Geometry: final body of the model. Coordinates: model frame, mm. A direction names the side the tool comes from. Give positions to 0.01 mm unless a question says otherwise; leave off trailing zeros. Write each loop counter-clockwise with the first axis right and the second up, starting at its lowest first coordinate (ties: lowest second). Pieces come first, ordered by that corner, then holes. Notation, with made-up numbers: (-7, 28) -> (23, 28) arc R35 ccw to (23, 62) -> close; hole circle Ø1 at (79.5, 1.25). An arc over 180 degrees is marked (long way). Answer as a JSON object with one key per item and string values.
from build123d import *

# Parameters (mm, degrees)
BOSS_EXTRUDE1_DEPTH      = 11
SKETCH2_W                = 60
SKETCH2_H                = 5
BOSS_EXTRUDE2_DEPTH      = 26
FILLET1_R                = 5
SKETCH4_R                = 1.75
CUT_EXTRUDE2_DEPTH       = 25
CUT_EXTRUDE3_DEPTH       = 25
FILLET1_OF_MIRROR1_R     = 5
CUT_EXTRUDE7_DEPTH       = 0.5
BOSS_EXTRUDE3_DEPTH      = 10
SKETCH20_R               = 1.95
CUT_EXTRUDE10_DEPTH      = 14
FILLET2_R                = 2
SKETCH21_W               = 5
SKETCH21_H               = 13
BOSS_EXTRUDE4_DEPTH      = 10
FILLET3_R                = 2
FILLET4_R                = 2
SKETCH24_W               = 27.361524014
SKETCH24_H               = 13
CUT_EXTRUDE12_DEPTH      = 5
SKETCH22_R               = 2.25
CUT_EXTRUDE11_DEPTH      = 38.361524014
CUT_EXTRUDE11_DEPTH_BACK = 3
SKETCH23_R               = 5.5
CUT_EXTRUDE13_DEPTH      = 5
BOSS_EXTRUDE5_DEPTH      = 3
FILLET5_R                = 2


with BuildPart() as part:
    # Sketch1 → Boss-Extrude1 (new body)
    with BuildSketch(Plane.XY):
        with BuildLine():
            Line((60, 35), (0, 35))
            Line((0, 35), (0, 40))
            ThreePointArc((0, 40), (-7.071067812, 37.071067812), (-10, 30))
            Line((-10, 30), (-10, 10))
            ThreePointArc((-10, 10), (-7.071067812, 2.928932188), (0, 0))
            Line((0, 0), (60, 0))
            ThreePointArc((60, 0), (67.071067812, 2.928932188), (70, 10))
            Line((70, 10), (70, 30))
            ThreePointArc((70, 30), (67.071067812, 37.071067812), (60, 40))
            Line((60, 40), (60, 35))
        make_face()
    extrude(amount=BOSS_EXTRUDE1_DEPTH)

    # Sketch2 → Boss-Extrude2 (add)
    with BuildSketch(Plane.XY.offset(11)):
        with Locations((30, 37.5)):
            Rectangle(SKETCH2_W, SKETCH2_H)
    boss_extrude2 = extrude(amount=-BOSS_EXTRUDE2_DEPTH)

    # Fillet1
    fillet1_edges = [part.edges().sort_by_distance(p)[0] for p in [
        (0, 37.5, -15),
        (60, 37.5, -15),
    ]]
    fillet(fillet1_edges, radius=FILLET1_R)

    # Sketch4 → Cut-Extrude2 (cut)
    with BuildSketch(Plane(origin=(0, 35, 0), x_dir=(-1, 0, 0), z_dir=(0, -1, 0))):
        with Locations((-55, 7.5)):
            Circle(SKETCH4_R)
        with Locations((-30, 7.5)):
            Circle(SKETCH4_R)
        with Locations((-5, 7.5)):
            Circle(SKETCH4_R)
    cut_extrude2 = extrude(amount=-CUT_EXTRUDE2_DEPTH, mode=Mode.SUBTRACT)

    # Sketch5 → Cut-Extrude3 (cut)
    with BuildSketch(Plane.XZ.offset(-35)):
        with BuildLine():
            Line((5, -14.75), (55, -14.75))
            ThreePointArc((55, -14.75), (58.358757211, -13.358757211), (59.75, -10))
            Line((59.75, -10), (59.75, -0.25))
            Line((59.75, -0.25), (59.75, 0))
            Line((59.75, 0), (60, 0))
            Line((60, 0), (60, -10))
            ThreePointArc((60, -10), (58.535533906, -13.535533906), (55, -15))
            Line((55, -15), (5, -15))
            ThreePointArc((5, -15), (1.464466094, -13.535533906), (0, -10))
            Line((0, -10), (0, 0))
            Line((0, 0), (0.25, 0))
            Line((0.25, 0), (0.25, -0.25))
            Line((0.25, -0.25), (0.25, -10))
            ThreePointArc((0.25, -10), (1.641242789, -13.358757211), (5, -14.75))
        make_face()
    extrude(amount=-CUT_EXTRUDE3_DEPTH, mode=Mode.SUBTRACT)

    # Mirror1: Boss-Extrude2, Cut-Extrude2 across plane
    add(boss_extrude2.mirror(Plane(origin=(0, 20, 0), x_dir=(0, 0, 1), z_dir=(0, -1, 0))))
    add(cut_extrude2.mirror(Plane(origin=(0, 20, 0), x_dir=(0, 0, 1), z_dir=(0, -1, 0))), mode=Mode.SUBTRACT)

    # Fillet1 of Mirror1
    fillet1_of_mirror1_edges = [part.edges().sort_by_distance(p)[0] for p in [
        (0, 2.5, -15),
        (60, 2.5, -15),
    ]]
    fillet(fillet1_of_mirror1_edges, radius=FILLET1_OF_MIRROR1_R)

    # Sketch16 → Cut-Extrude7 (cut)
    with BuildSketch(Plane.XZ.offset(-35)):
        with BuildLine():
            Line((0.25, 0), (0.25, -10))
            ThreePointArc((0.25, -10), (1.641242789, -13.358757211), (5, -14.75))
            Line((5, -14.75), (55, -14.75))
            ThreePointArc((55, -14.75), (58.358757211, -13.358757211), (59.75, -10))
            Line((59.75, -10), (59.75, 0))
            Line((59.75, 0), (0.25, 0))
        make_face()
    extrude(amount=-CUT_EXTRUDE7_DEPTH, mode=Mode.SUBTRACT)

    # Sketch19 → Boss-Extrude3 (add)
    with BuildSketch(Plane.XY.offset(11)):
        with BuildLine():
            Line((-10, 13), (15, 13))
            Line((15, 13), (15, 9.995431427))
            ThreePointArc((15, 9.995431427), (14.414213562, 8.581217864), (13, 7.995431427))
            Line((13, 7.995431427), (0, 7.995431427))
            Line((0, 7.995431427), (0, 5.995431427))
            Line((0, 5.995431427), (15, 5.995431427))
            ThreePointArc((15, 5.995431427), (16.414213562, 6.581217864), (17, 7.995431427))
            Line((17, 7.995431427), (17, 13))
            Line((17, 13), (22, 13))
            Line((22, 13), (22, 0))
            Line((22, 0), (0, 0))
            ThreePointArc((0, 0), (-7.071067812, 2.928932188), (-10, 10))
            Line((-10, 10), (-10, 13))
        make_face()
    extrude(amount=BOSS_EXTRUDE3_DEPTH)

    # Sketch20 → Cut-Extrude10 (cut)
    with BuildSketch(Plane(origin=(0, 0, 0), x_dir=(-1, 0, 0), z_dir=(0, -1, 0))):
        with Locations((-8.068741, -16)):
            Circle(SKETCH20_R)
    extrude(amount=-CUT_EXTRUDE10_DEPTH, mode=Mode.SUBTRACT)

    # Fillet2
    fillet2_edges = [part.edges().sort_by_distance(p)[0] for p in [
        (15, 13, 16),
    ]]
    fillet(fillet2_edges, radius=FILLET2_R)

    # Sketch21 → Boss-Extrude4 (add)
    with BuildSketch(Plane.XY.offset(11)):
        with BuildLine():
            Line((70, 13), (60, 13))
            Line((60, 13), (60, 0))
            ThreePointArc((60, 0), (67.071067812, 2.928932188), (70, 10))
            Line((70, 10), (70, 13))
        make_face()
        with Locations((30.138475986, 6.5)):
            Rectangle(SKETCH21_W, SKETCH21_H)
    extrude(amount=BOSS_EXTRUDE4_DEPTH)

    # Fillet3
    fillet3_edges = [part.edges().sort_by_distance(p)[0] for p in [
        (27.638475986, 13, 16),
    ]]
    fillet(fillet3_edges, radius=FILLET3_R)

    # Fillet4
    fillet4_edges = [part.edges().sort_by_distance(p)[0] for p in [
        (27.638475986, 0, 16),
    ]]
    fillet(fillet4_edges, radius=FILLET4_R)

    # Sketch24 → Cut-Extrude12 (cut)
    with BuildSketch(Plane.XY.offset(11)):
        with Locations((46.319237993, 6.5)):
            Rectangle(SKETCH24_W, SKETCH24_H)
    extrude(amount=-CUT_EXTRUDE12_DEPTH, mode=Mode.SUBTRACT)

    # Sketch22 → Cut-Extrude11 (cut, two sides)
    with BuildSketch(Plane(origin=(32.638475986, 0, 0), x_dir=(0, 0, -1), z_dir=(1, 0, 0))) as cut_extrude11_sk:
        with Locations((-12, 6.5)):
            Circle(SKETCH22_R)
    extrude(amount=CUT_EXTRUDE11_DEPTH, mode=Mode.SUBTRACT)
    extrude(cut_extrude11_sk.sketch, amount=-CUT_EXTRUDE11_DEPTH_BACK, mode=Mode.SUBTRACT)

    # Sketch23 → Cut-Extrude13 (cut)
    with BuildSketch(Plane(origin=(70, 0, 0), x_dir=(0, 0, -1), z_dir=(1, 0, 0))):
        with Locations((-12, 6.5)):
            Circle(SKETCH23_R)
    extrude(amount=-CUT_EXTRUDE13_DEPTH, mode=Mode.SUBTRACT)

    # Sketch25 → Boss-Extrude5 (add)
    with BuildSketch(Plane.XY.offset(21)):
        with BuildLine():
            Line((60, 0), (32.638475986, 0))
            Line((32.638475986, 0), (29.638475986, 0))
            ThreePointArc((29.638475986, 0), (28.224262424, 0.585786438), (27.638475986, 2))
            Line((27.638475986, 2), (27.638475986, 11))
            ThreePointArc((27.638475986, 11), (28.224262424, 12.414213562), (29.638475986, 13))
            Line((29.638475986, 13), (32.638475986, 13))
            Line((32.638475986, 13), (60, 13))
            Line((60, 13), (70, 13))
            Line((70, 13), (70, 10))
            ThreePointArc((70, 10), (67.071067812, 2.928932188), (60, 0))
        make_face()
    extrude(amount=-BOSS_EXTRUDE5_DEPTH)

    # Fillet5
    fillet5_edges = [part.edges().sort_by_distance(p)[0] for p in [
        (22, 0, 16),
        (22, 13, 16),
    ]]
    fillet(fillet5_edges, radius=FILLET5_R)


solid = part.part
Q1. Mould query, pull axis Z, two halves, no side actions, for faces 4 (the flat face through (0.25, 38, -5)), 5 (the cylindrical face through (62.46, 8.02, 13.66)), 6 (the flat face through (6, 5, 21)). Classes: pulls with the +Z half, pulls with the -Z half, needs draft (parallel to the pull), parting line crosses it, or undercut.
Values:
{"face 4": "needs draft", "face 5": "undercut", "face 6": "pulls with the +Z half"}
Q2. Cut plane A-A (z = -7.5). State how many separate pieces and enclosed holes the cut face has, and give its area (3 significant figures).
Values:
{"separate pieces": "8", "enclosed holes": "0", "area": "468 mm²"}
Q3. Material intervals for L1, parallel to X at y = 10.5, z = 13.5; L2, parallel to X at y = 38.25, z = -7.5; L3, parallel to Y at x = 24, z = -11.5, sorted ascending. Write a range as from..to.
Values:
{"L1": "-10..15, 17..22, 27.64..32.64, 60..65", "L2": "0.25..3.25, 6.75..28.25, 31.75..53.25, 56.75..59.75", "L3": "0..5, 35.5..40"}
Q4. Cut plane B-B (x = 45). Return the cut outline in (y, z), and give its area (3 significant figures).
Values:
{"outline": "(0, -15) -> (5, -15) -> (5, 0) -> (35.5, 0) -> (35.5, -14.75) -> (40, -14.75) -> (40, 11) -> (13, 11) -> (13, 6) -> (0, 6) -> close; (0, 18) -> (13, 18) -> (13, 21) -> (0, 21) -> close", "area": "555 mm²"}
Q5. Set-up query: faces 1 (the cylindrical face through (14.4, 12.43, 16.07)), 2 (the flat face through (46, 13, 9)), 3 (the flat face through (5, 7.995, 16)). Return all of +Z, -Z, +X, -X, +Y, -Y with unobstructed straight access to the full face (end or side cutting, diameter ignored); none if empty.
Values:
{"face 1": "+Z, +Y", "face 2": "-Y", "face 3": "+Z"}
Q6. Cut plane C-C (y = 38). Return the cut outline in (x, z), and give its area (3 significant figures).
Values:
{"outline": "(-6, 0) -> (0.25, 0) -> (0.25, -10) arc R4.75 ccw to (5, -14.75) -> (55, -14.75) arc R4.75 ccw to (59.75, -10) -> (59.75, 0) -> (66, 0) -> (66, 11) -> (-6, 11) -> close; hole circle Ø3.5 at (5, -7.5); hole circle Ø3.5 at (30, -7.5); hole circle Ø3.5 at (55, -7.5)", "area": "1,630 mm²"}
Q7. First-contact query: P1, Ø3, axis at y = 8.5, z = 12, coming from the +X side; P2, Ø4, axis at y = 6.5, z = 12, coming from the +X side; P3, Ø1.3, axis at y = 38.5, z = -7, coming from the -X side. Flat tips, straight axial feed; report the tip coordinate or a pass-through.
Values:
{"P1": "x = 65", "P2": "x = 29.64", "P3": "x = 0.25"}
Q8. Cut plane D-D (z = -1). Return the cut outline in (x, y).
Values:
{"outline": "(0, 0) -> (60, 0) -> (60, 5) -> (0, 5) -> close; (0.25, 35.5) -> (59.75, 35.5) -> (59.75, 40) -> (0.25, 40) -> close"}
